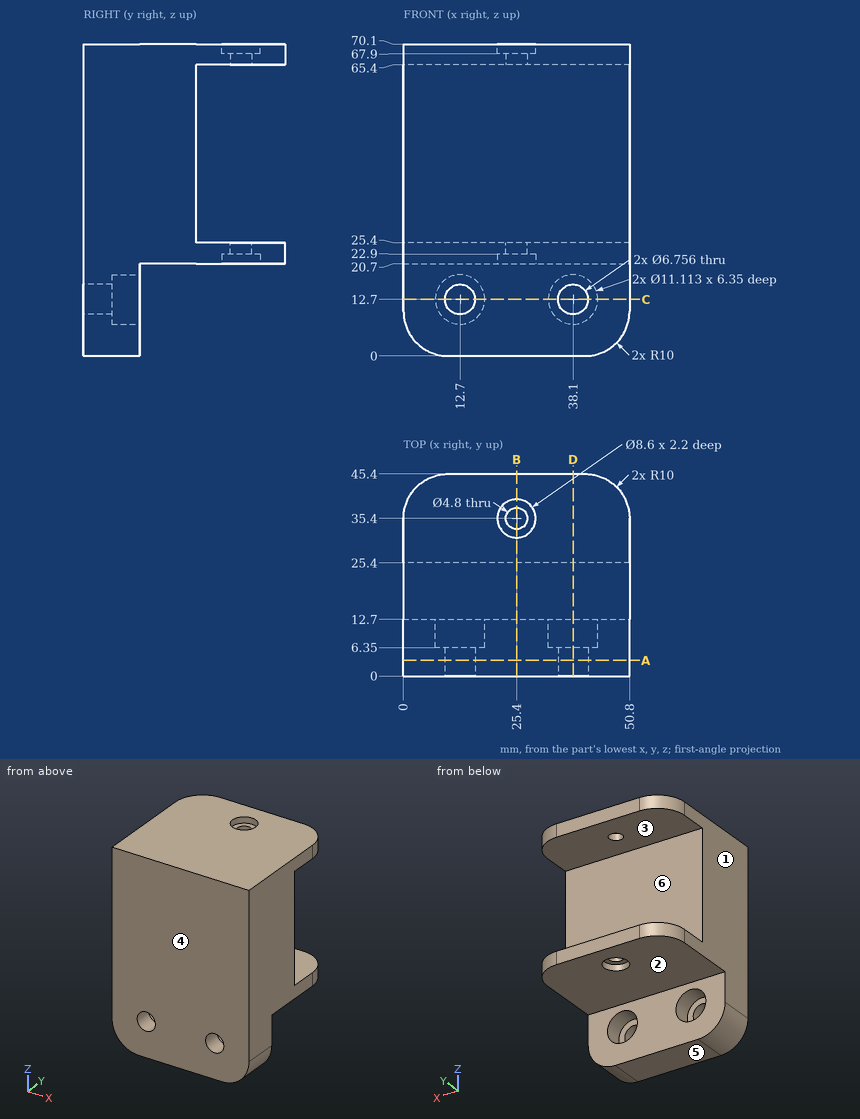
Verification items for this drawing (mm, ordinates from the low corner). A direction names the side the tool comes from. Round coordinates to 2 decimals unless told otherwise and drop trailing zeros. Loops run counter-clockwise (first coordinate to the right, second up) from the corner with the lowest first, then second, coordinate; pieces in that order, holes last. Notation, with made-up numbers: (-34.75, -34.5) -> (-20.75, -34.5) arc R26 ccw to (-20.75, 2.5) -> close; hole circle Ø5 at (30.25, 64). An arc over 180 degrees is marked (long way). Write item = value, one per line. Start each with the question number.
1) Release check for a two-part mould opening along Z. For the marked faces 4, 5 and 6 record: released by +Z, released by -Z, zero draft, split by the parting line, or undercut.
2) Thickness scan on probe 1 along Z at (x, y) = (38, 4); probe 2 along Z at (x, y) = (23.5, 43.5); probe 3 along X at (y, z) = (35, 21). Record the ranges inside material, lowest first.
3) Sectioned sample at A-A, the plane y = 3.5. Record the cut outline in (x, z), plus the area to 3 significant figures.
4) Sectioned sample at C-C, the plane z = 12.7. Record the cut outline in (x, y), plus the area to 3 significant figures.
5) Sectioned sample at D-D, the plane x = 38.1. Record the cut outline in (y, z), plus the area to 3 significant figures.
6) Set-up check for the marked faces 1, 2 and 3: record each of +Z, -Z, +X, -X, +Y, -Y from which the full face is reachable in a straight line by a thin tool's end or side.
7) Gauge pin test, flat ends, axial feed: pin 1 Ø9 at (x, z) = (12.7, 12.7) entering from +Y; pin 2 Ø2.5 at (x, y) = (23.5, 34.5) entering from -Z; pin 3 Ø6 at (x, y) = (32, 33) entering from -Z. Record the tip position at first contact, or that the pin passes through.
8) Sectioned sample at B-B, the plane x = 25.4. Record the cut outline in (y, z).
Results are:
q1.face_4 = zero draft
q1.face_5 = released by -Z
q1.face_6 = undercut
q2.probe_1 = 0 to 9.32, 16.08 to 70.1
q2.probe_2 = 20.7 to 25.4, 65.4 to 70.1
q2.probe_3 = 0 to 21.12, 29.68 to 50.8
q3.outline = (0, 10) arc R10 ccw to (10, 0) -> (40.8, 0) arc R10 ccw to (50.8, 10) -> (50.8, 70.1) -> (0, 70.1) -> close; hole circle Ø6.76 at (12.7, 12.7); hole circle Ø6.76 at (38.1, 12.7)
q3.area = 3,450 mm^2
q4.outline = (0, 0) -> (9.32, 0) -> (9.32, 6.35) -> (7.14, 6.35) -> (7.14, 12.7) -> (0, 12.7) -> close; (16.08, 0) -> (34.72, 0) -> (34.72, 6.35) -> (32.54, 6.35) -> (32.54, 12.7) -> (18.26, 12.7) -> (18.26, 6.35) -> (16.08, 6.35) -> close; (41.48, 0) -> (50.8, 0) -> (50.8, 12.7) -> (43.66, 12.7) -> (43.66, 6.35) -> (41.48, 6.35) -> close
q4.area = 418 mm^2
q5.outline = (0, 0) -> (12.7, 0) -> (12.7, 7.14) -> (6.35, 7.14) -> (6.35, 9.32) -> (0, 9.32) -> close; (0, 16.08) -> (6.35, 16.08) -> (6.35, 18.26) -> (12.7, 18.26) -> (12.7, 20.7) -> (45.4, 20.7) -> (45.4, 25.4) -> (25.4, 25.4) -> (25.4, 65.4) -> (45.4, 65.4) -> (45.4, 70.1) -> (0, 70.1) -> close
q5.area = 1,590 mm^2
q6.face_1 = +Z, -Z, -X, +Y, -Y
q6.face_2 = -Z, +X, -X, +Y
q6.face_3 = +X, -X, +Y
q7.pin_1 = 6.35
q7.pin_2 = 22.9
q7.pin_3 = 20.7
q8.outline = (0, 0) -> (12.7, 0) -> (12.7, 20.7) -> (31.1, 20.7) -> (31.1, 22.9) -> (33, 22.9) -> (33, 25.4) -> (25.4, 25.4) -> (25.4, 65.4) -> (33, 65.4) -> (33, 67.9) -> (31.1, 67.9) -> (31.1, 70.1) -> (0, 70.1) -> close; (37.8, 22.9) -> (39.7, 22.9) -> (39.7, 20.7) -> (45.4, 20.7) -> (45.4, 25.4) -> (37.8, 25.4) -> close; (37.8, 65.4) -> (45.4, 65.4) -> (45.4, 70.1) -> (39.7, 70.1) -> (39.7, 67.9) -> (37.8, 67.9) -> close
